CAD build for the part. Positions are in the model's coordinates, mm. A direction names the side the tool comes from. Give positions to 0.01 mm unless a question says otherwise; leave off trailing zeros. Write each loop counter-clockwise with the first axis right and the second up, starting at its lowest first coordinate (ties: lowest second). Pieces come first, ordered by that corner, then holes. Notation, with made-up numbers: (-29, 33.5) - (-20, 33.5) arc R12 cw to (-20, 44.5) - close; hole circle Ø3 at (38.25, 52). An arc over 180 degrees is marked (long way). Answer as a JSON object with one key per item and string values.
from build123d import *

# Parameters (mm, degrees)
SKETCH_1_W           = 97.5
SKETCH_1_H           = 19.5
EXTRUDE_1_DEPTH      = 20
SKETCH_2_W           = 29.8652771
SKETCH_2_H           = 10
CUT_EXTRUDE_4_DEPTH  = 29
SKETCH_3_W           = 10
SKETCH_3_H           = 10
CUT_EXTRUDE_5_DEPTH  = 10
SKETCH_4_W           = 19.8652771
SKETCH_4_H           = 10
CUT_EXTRUDE_6_DEPTH  = 10
SKETCH_5_W           = 10
SKETCH_5_H           = 10
CUT_EXTRUDE_7_DEPTH  = 10
SHELL_1_T            = -2
SKETCH_7_W           = 10
SKETCH_7_H           = 10
CUT_EXTRUDE_8_DEPTH  = 10
SKETCH_8_W           = 10.001998353
SKETCH_8_H           = 10
CUT_EXTRUDE_9_DEPTH  = 10
SKETCH_9_W           = 10
SKETCH_9_H           = 10
EXTRUDE_3_DEPTH      = 10
SKETCH_10_W          = 8.5
SKETCH_10_H          = 8.69149108
EXTRUDE_4_DEPTH      = 0.5
SKETCH_11_W          = 8
SKETCH_11_H          = 8
EXTRUDE_5_DEPTH      = 0.5
SKETCH_15_W          = 10.5
SKETCH_15_H          = 0.69149108
EXTRUDE_18_DEPTH     = 9.5
SKETCH_18_W          = 8
SKETCH_18_H          = 8
EXTRUDE_22_DEPTH     = 0.5
SKETCH_21_W          = 10
SKETCH_21_H          = 0.094242597
EXTRUDE_25_DEPTH     = 10.5
SKETCH_23_W          = 20
SKETCH_23_H          = 10
EXTRUDE_27_DEPTH     = 10
SKETCH_24_W          = 10.001998353
SKETCH_24_H          = 10
EXTRUDE_28_DEPTH     = 10
SKETCH_25_W          = 9.8
SKETCH_25_H          = 10
EXTRUDE_29_DEPTH     = 10
SKETCH_31_W          = 10
SKETCH_31_H          = 0.5
CUT_EXTRUDE_11_DEPTH = 11.5
SKETCH_32_W          = 16
SKETCH_32_H          = 15.5
EXTRUDE_43_DEPTH     = 0.5


with BuildPart() as part:
    # 草圖1 → 填料-伸長1 (new body)
    with BuildSketch(Plane.XY):
        Rectangle(SKETCH_1_W, SKETCH_1_H)
    extrude(amount=EXTRUDE_1_DEPTH)

    # 草圖2 → 除料-伸長4 (cut)
    with BuildSketch(Plane(origin=(0, 9.75, 0), x_dir=(1, 0, 0), z_dir=(0, 1, 0))):
        with Locations((-5.06736145, -15)):
            Rectangle(SKETCH_2_W, SKETCH_2_H)
    extrude(amount=-CUT_EXTRUDE_4_DEPTH, mode=Mode.SUBTRACT)

    # 草圖3 → 除料-伸長5 (cut)
    with BuildSketch(Plane(origin=(0, 9.75, 0), x_dir=(1, 0, 0), z_dir=(0, 1, 0))):
        with Locations((14.8652771, -15)):
            Rectangle(SKETCH_3_W, SKETCH_3_H)
    extrude(amount=-CUT_EXTRUDE_5_DEPTH, mode=Mode.SUBTRACT)

    # 草圖4 → 除料-伸長6 (cut)
    with BuildSketch(Plane(origin=(0, 9.75, 0), x_dir=(1, 0, 0), z_dir=(0, 1, 0))):
        with Locations((9.93263855, -5)):
            Rectangle(SKETCH_4_W, SKETCH_4_H)
    extrude(amount=-CUT_EXTRUDE_6_DEPTH, mode=Mode.SUBTRACT)

    # 草圖5 → 除料-伸長7 (cut)
    with BuildSketch(Plane(origin=(0, 9.75, 0), x_dir=(1, 0, 0), z_dir=(0, 1, 0))):
        with Locations((-5, -5)):
            Rectangle(SKETCH_5_W, SKETCH_5_H)
    extrude(amount=-CUT_EXTRUDE_7_DEPTH, mode=Mode.SUBTRACT)

    # 薄殼1
    shell_1_openings = [part.faces().sort_by_distance(p)[0] for p in [
        (48.75, 0, 10),
    ]]
    offset(amount=SHELL_1_T, openings=shell_1_openings, kind=Kind.INTERSECTION)

    # 草圖7 → 除料-伸長8 (cut)
    with BuildSketch(Plane(origin=(0, 9.75, 0), x_dir=(1, 0, 0), z_dir=(0, 1, 0))):
        with Locations((-15, -5)):
            Rectangle(SKETCH_7_W, SKETCH_7_H)
    extrude(amount=-CUT_EXTRUDE_8_DEPTH, mode=Mode.SUBTRACT)

    # 草圖8 → 除料-伸長9 (cut)
    with BuildSketch(Plane(origin=(0, 9.75, 0), x_dir=(1, 0, 0), z_dir=(0, 1, 0))):
        with Locations((-25.000999177, -15)):
            Rectangle(SKETCH_8_W, SKETCH_8_H)
    extrude(amount=-CUT_EXTRUDE_9_DEPTH, mode=Mode.SUBTRACT)

    # 草圖9 → 填料-伸長3 (add)
    with BuildSketch(Plane(origin=(0, -0.25, 0), x_dir=(1, 0, 0), z_dir=(0, 1, 0))):
        with Locations((4.8652771, -15)):
            Rectangle(SKETCH_9_W, SKETCH_9_H)
    extrude(amount=-EXTRUDE_3_DEPTH)

    # 草圖10 → 填料-伸長4 (add)
    with BuildSketch(Plane(origin=(0, -0.25, 0), x_dir=(1, 0, 0), z_dir=(0, 1, 0))):
        with Locations((-26.25, -13.65425446)):
            Rectangle(SKETCH_10_W, SKETCH_10_H)
    extrude(amount=-EXTRUDE_4_DEPTH)

    # 草圖11 → 填料-伸長5 (add)
    with BuildSketch(Plane(origin=(-30.001998353, 0, 0), x_dir=(0, 0, -1), z_dir=(1, 0, 0))):
        with Locations((-14, 3.75)):
            Rectangle(SKETCH_11_W, SKETCH_11_H)
    extrude(amount=-EXTRUDE_5_DEPTH)

    # 草圖15 → 填料-伸長18 (add)
    with BuildSketch(Plane(origin=(0, -0.25, 0), x_dir=(1, 0, 0), z_dir=(0, 1, 0))):
        with Locations((-25.25, -9.65425446)):
            Rectangle(SKETCH_15_W, SKETCH_15_H)
    extrude(amount=EXTRUDE_18_DEPTH)

    # 草圖18 → 填料-伸長22 (add)
    with BuildSketch(Plane(origin=(0, -0.25, 0), x_dir=(1, 0, 0), z_dir=(0, 1, 0))):
        with Locations((-16, -6)):
            Rectangle(SKETCH_18_W, SKETCH_18_H)
    extrude(amount=-EXTRUDE_22_DEPTH)

    # 草圖21 → 填料-伸長25 (add)
    with BuildSketch(Plane(origin=(-20, 0, 0), x_dir=(0, 0, -1), z_dir=(1, 0, 0))):
        with Locations((-5, -0.297121299)):
            Rectangle(SKETCH_21_W, SKETCH_21_H)
    extrude(amount=EXTRUDE_25_DEPTH)

    # 草圖23 → 填料-伸長27 (add)
    with BuildSketch(Plane.ZY.offset(-19.8652771)):
        with Locations((10, 4.75)):
            Rectangle(SKETCH_23_W, SKETCH_23_H)
    extrude(amount=EXTRUDE_27_DEPTH)

    # 草圖24 → 填料-伸長28 (add)
    with BuildSketch(Plane(origin=(0, -0.25, 0), x_dir=(1, 0, 0), z_dir=(0, 1, 0))):
        with Locations((-25.000999177, -15)):
            Rectangle(SKETCH_24_W, SKETCH_24_H)
    extrude(amount=EXTRUDE_28_DEPTH)

    # 草圖25 → 填料-伸長29 (add)
    with BuildSketch(Plane(origin=(0, -0.25, 0), x_dir=(1, 0, 0), z_dir=(0, 1, 0))):
        with Locations((-15.1, -5)):
            Rectangle(SKETCH_25_W, SKETCH_25_H)
    extrude(amount=EXTRUDE_29_DEPTH)

    # 草圖31 → 除料-伸長11 (cut)
    with BuildSketch(Plane(origin=(9.8652771, 0, 0), x_dir=(0, 0, -1), z_dir=(1, 0, 0))):
        with Locations((-15, -10)):
            Rectangle(SKETCH_31_W, SKETCH_31_H)
    extrude(amount=-CUT_EXTRUDE_11_DEPTH, mode=Mode.SUBTRACT)

    # 草圖32 → 填料-伸長43 (add)
    with BuildSketch(Plane(origin=(48.75, 0, 0), x_dir=(0, 0, -1), z_dir=(1, 0, 0))):
        with Locations((-10, 0)):
            Rectangle(SKETCH_32_W, SKETCH_32_H)
    extrude(amount=-EXTRUDE_43_DEPTH)


solid = part.part
(1) Saw through at D-D, the plane y = -5.25. Give the cut face in (x, z).
Answer key:
{"outline": "(-48.75, 0) - (48.75, 0) - (48.75, 20) - (-0.13, 20) - (-0.13, 10) - (-20, 10) - (-20, 20) - (-48.75, 20) - close; hole (-46.75, 2) - (48.25, 2) - (48.25, 18) - (11.87, 18) - (11.87, 8) - (-22, 8) - (-22, 18) - (-46.75, 18) - close"}
(2) 3-axis set-ups, long thin cutter, end or side, ignore diameter. For faces 4 (the face through (-30.502, 4, 14)), 5 (the face through (2, -0.25, 8)), 6 (the face through (-0.135, -5, 15)), 7 (the face through (-30, 9.75, 10)): which of +Z, -Z, +X, -X, +Y, -Y reach the whole face in a straight line?
Answer key:
{"face 4": "none", "face 5": "+Z, -Z, +Y", "face 6": "+Z, +Y, -Y", "face 7": "+Z, -Z, +X, -X, +Y"}
(3) Saw through at C-C, the plane x = 35. Give the cut face in (y, z), and give its area (3 significant figures).
Answer key:
{"outline": "(-9.75, 0) - (9.75, 0) - (9.75, 20) - (-9.75, 20) - close; hole (-7.75, 2) - (7.75, 2) - (7.75, 18) - (-7.75, 18) - close", "area": "142 mm²"}
(4) Saw through at A-A, the plane y = 3. State how many separate pieces and enclosed holes the cut face has, and give its area (3 significant figures).
Answer key:
{"separate pieces": "2", "enclosed holes": "2", "area": "694 mm²"}
(5) Probe L1, parallel to X at y = 0, z = 3.75; L2, parallel to X at y = 3.5, z = 15; L3, parallel to Y at x = -36, z = 4. List the from-to ranges inside material, lowest first. Write a range as [from, to].
Answer key:
{"L1": "x = [-48.75, -46.75], [-20, -10.2], [9.87, 21.87], [48.25, 48.75]", "L2": "x = [-48.75, -46.75], [-30.5, -20], [9.87, 21.87], [48.25, 48.75]", "L3": "y = [-9.75, -7.75], [7.75, 9.75]"}
(6) Pull direction X, two halves, no side cores. Call faces 1 (the face through (0, -7.75, 6)), 2 (the face through (-35, 0, 20)), 3 (the face through (-48.75, 0, 10)): pulls with the +X half, pulls with the -X half, needs draft (parallel to the pull), parting line crosses it, or undercut.
Answer key:
{"face 1": "undercut", "face 2": "needs draft", "face 3": "pulls with the -X half"}
